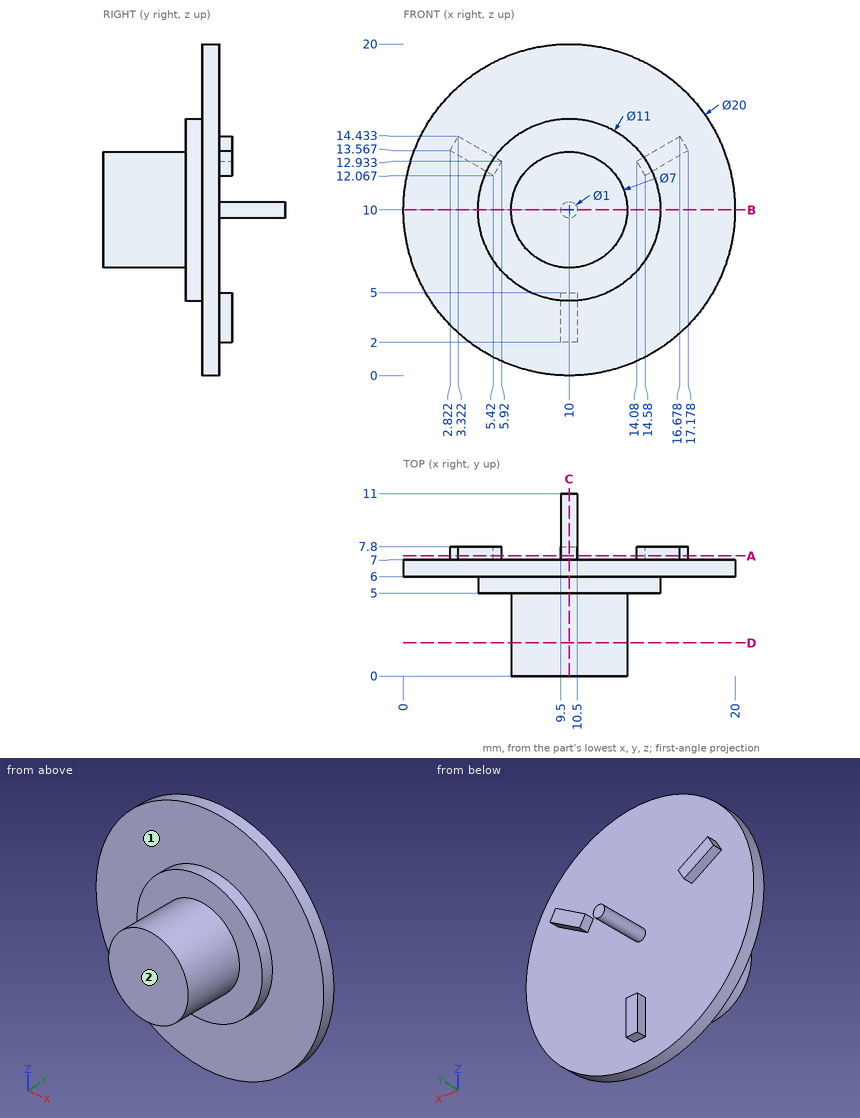
The drawing under review shows one solid part. Ordinate dimensions are in mm from its lowest x, y, z. A direction names the side the tool comes from. Coordinates: 2 decimals unless noted, no trailing zeros. Loops run counter-clockwise (first coordinate to the right, second up) from the corner with the lowest first, then second, coordinate; pieces in that order, holes last.
Item 1: Add section B-B (z = 10). Write out the cut boundary in (x, y).
Completed:
outline: (0, 6) - (4.5, 6) - (4.5, 5) - (6.5, 5) - (6.5, 0) - (13.5, 0) - (13.5, 5) - (15.5, 5) - (15.5, 6) - (20, 6) - (20, 7) - (10.5, 7) - (10.5, 11) - (9.5, 11) - (9.5, 7) - (0, 7) - close
Item 2: Clearance check with flat-ended pins moving along their axes: pin 1 (0.9 mm diameter, centred on y = 7, z = 3, fed in from -X); pin 2 (0.7 mm diameter, centred on x = 3.5, z = 13.5, fed in from +Y); pin 3 (9 mm diameter, centred on x = 11.5, z = 7.5, fed in from -Y); pin 4 (6 mm diameter, centred on x = 15.5, y = 8.5, fed in from +Z). State where each tip first meets the part, or that it passes through.
Completed:
pin 1: stops at x = 2.44
pin 2: stops at y = 7.8
pin 3: stops at y = 0
pin 4: stops at z = 19.57
Item 3: Add section D-D (y = 2). Write out the cut boundary in (x, z), and give its area (3 significant figures).
Completed:
outline: circle Ø7 at (10, 10)
area: 38.5 mm2
Item 4: For the marked faces 1 and 2, list the 3-axis set-ups (+Z, -Z, +X, -X, +Y, -Y) from which the entire face can be reached by the end or side of a thin tool; tool diameter is ignored.
Completed:
face 1: -Y
face 2: +Z, -Z, +X, -X, -Y
Item 5: Wall thickness on L1, parallel to Y at x = 6.25, z = 12.5; L2, parallel to Y at x = 15.5, z = 17.5; L3, parallel to Z at x = 9.5, y = 4: over which ranges is each line inside the solid? List them lowest first.
Completed:
L1: y = 5 to 7
L2: y = 6 to 7
L3: z = 6.54 to 13.46
Item 6: Add section A-A (y = 7.25). Write out the cut boundary in (x, z).
Completed:
outline: (2.82, 13.57) - (5.42, 12.07) - (5.92, 12.93) - (3.32, 14.43) - close; (9.5, 2) - (10.5, 2) - (10.5, 5) - (9.5, 5) - close; circle Ø1 at (10, 10); (14.08, 12.93) - (14.58, 12.07) - (17.18, 13.57) - (16.68, 14.43) - close
Item 7: Add section C-C (x = 10). Write out the cut boundary in (y, z).
Completed:
outline: (0, 6.5) - (5, 6.5) - (5, 4.5) - (6, 4.5) - (6, 0) - (7, 0) - (7, 2) - (7.8, 2) - (7.8, 5) - (7, 5) - (7, 9.5) - (11, 9.5) - (11, 10.5) - (7, 10.5) - (7, 20) - (6, 20) - (6, 15.5) - (5, 15.5) - (5, 13.5) - (0, 13.5) - close
